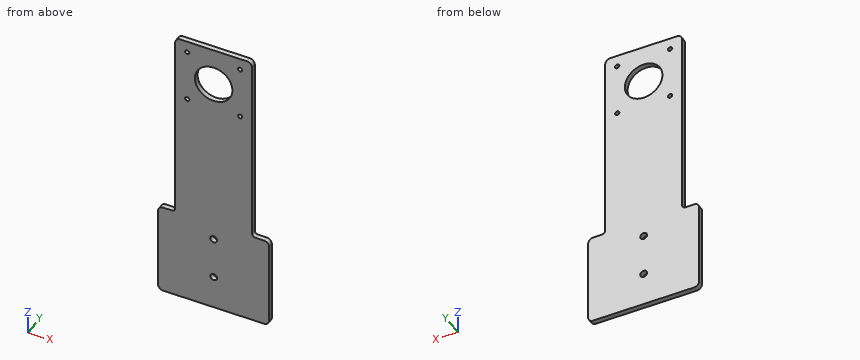
```python
from build123d import *

# Parameters (mm, degrees)
SKETCH1_R           = 2
SKETCH1_R_2         = 1.25
SKETCH1_R_3         = 11
BOSS_EXTRUDE1_DEPTH = 3
FILLET1_R           = 3
FILLET2_R           = 3
FILLET3_R           = 3
FILLET4_R           = 3
FILLET5_R           = 3
FILLET7_R           = 3
FILLET8_R           = 2
FILLET9_R           = 2


with BuildPart() as part:
    # Sketch1 → Boss-Extrude1 (new body)
    with BuildSketch(Plane(origin=(0, 0, 0), x_dir=(1, 0, 0), z_dir=(0, 1, 0))):
        Polygon((0, 111.61362417), (-32.5, 111.61362417), (-32.5, 56.61362417), (-22.5, 56.61362417), (-22.5, -58.38637583), (0, -58.38637583), (22.5, -58.38637583), (22.5, 56.61362417), (32.5, 56.61362417), (32.5, 111.61362417), align=None)
        with Locations(Location((0, 91.61362417, 0), (0, 0, 270))):
            Circle(SKETCH1_R, mode=Mode.SUBTRACT)
        with Locations(Location((0, 66.61362417, 0), (0, 0, 270))):
            Circle(SKETCH1_R, mode=Mode.SUBTRACT)
        with Locations(Location((-15.5, -20.454039675, 0), (0, 0, 270))):
            Circle(SKETCH1_R_2, mode=Mode.SUBTRACT)
        with Locations(Location((-15.5, -51.454039675, 0), (0, 0, 270))):
            Circle(SKETCH1_R_2, mode=Mode.SUBTRACT)
        with Locations(Location((15.5, -51.454039675, 0), (0, 0, 270))):
            Circle(SKETCH1_R_2, mode=Mode.SUBTRACT)
        with Locations(Location((15.5, -20.454039675, 0), (0, 0, 270))):
            Circle(SKETCH1_R_2, mode=Mode.SUBTRACT)
        with Locations(Location((0, -35.954039675, 0), (0, 0, 270))):
            Circle(SKETCH1_R_3, mode=Mode.SUBTRACT)
    extrude(amount=BOSS_EXTRUDE1_DEPTH)

    # Fillet1
    fillet1_edges = [part.edges().sort_by_distance(p)[0] for p in [
        (32.5, 1.5, -111.61362417),
    ]]
    fillet(fillet1_edges, radius=FILLET1_R)

    # Fillet2
    fillet2_edges = [part.edges().sort_by_distance(p)[0] for p in [
        (-32.5, 1.5, -111.61362417),
    ]]
    fillet(fillet2_edges, radius=FILLET2_R)

    # Fillet3
    fillet3_edges = [part.edges().sort_by_distance(p)[0] for p in [
        (-32.5, 1.5, -56.61362417),
    ]]
    fillet(fillet3_edges, radius=FILLET3_R)

    # Fillet4
    fillet4_edges = [part.edges().sort_by_distance(p)[0] for p in [
        (32.5, 1.5, -56.61362417),
    ]]
    fillet(fillet4_edges, radius=FILLET4_R)

    # Fillet5
    fillet5_edges = [part.edges().sort_by_distance(p)[0] for p in [
        (22.5, 1.5, 58.38637583),
    ]]
    fillet(fillet5_edges, radius=FILLET5_R)

    # Fillet7
    fillet7_edges = [part.edges().sort_by_distance(p)[0] for p in [
        (-22.5, 1.5, 58.38637583),
    ]]
    fillet(fillet7_edges, radius=FILLET7_R)

    # Fillet8
    fillet8_edges = [part.edges().sort_by_distance(p)[0] for p in [
        (-22.5, 1.5, -56.61362417),
    ]]
    fillet(fillet8_edges, radius=FILLET8_R)

    # Fillet9
    fillet9_edges = [part.edges().sort_by_distance(p)[0] for p in [
        (22.5, 1.5, -56.61362417),
    ]]
    fillet(fillet9_edges, radius=FILLET9_R)


solid = part.part
```
Here's how the part is built. I have some questions about the finished solid (model axes, mm). Coordinates: 2 decimals unless noted, no trailing zeros. Order: outer loops, then holes, each group sorted by start corner. A loop starts at its lowest first (then second) coordinate and runs counter-clockwise, first axis right, second up. Notation, with made-up numbers: M 50.25,54 L 96.25,54 A28 cw 96.25,76 Z; hole C 11,40.5 d3. An arc over 180 degrees is marked long. Answer as a JSON object with one key per item and string values. Group by question number.
(1) Suppose I cut it at B-B, the plane y = 0.9. Please give me the cut outline in (x, z), then the cut area to 3 significant figures.
(2) Suppose I cut it at A-A, the plane x = 0. Please give me the cut outline in (y, z), then the cut area to 3 significant figures.
(3) Suppose I cut it at C-C, the plane z = -22.5. Please give me the cut outline in (x, y).
(4) Suppose I cut it at D-D, the plane x = -26.5. Please give me the cut outline in (y, z).
(5) For pin 1 (5 mm diameter, centred on x = 21, z = -89, fed in from -Y); pin 2 (1.5 mm diameter, centred on y = 1, z = -41, fed in from +X); pin 3 (0.9 mm diameter, centred on x = -26, y = 1.5, fed in from +Z), each with a flat end and sliding along its axis, tell me the tip position at first contact or that it passes through.
(6) I need wall thicknesses on probe 1 along X at (y, z) = (0.65, 20.5); probe 2 along Z at (x, y) = (14.5, 1.05); probe 3 along X at (y, z) = (2.8, 52). Which ranges of each line are inside material? Lowest first, please.
Values found:
{
 "1": {"outline": "M -32.5,-108.61 A3 ccw -29.5,-111.61 L 29.5,-111.61 A3 ccw 32.5,-108.61 L 32.5,-59.61 A3 ccw 29.5,-56.61 L 24.5,-56.61 A2 cw 22.5,-54.61 L 22.5,55.39 A3 ccw 19.5,58.39 L -19.5,58.39 A3 ccw -22.5,55.39 L -22.5,-54.61 A2 cw -24.5,-56.61 L -29.5,-56.61 A3 ccw -32.5,-59.61 Z; hole C -15.5,20.45 d2.5; hole C -15.5,51.45 d2.5; hole C 0,35.95 d22; hole C 0,-91.61 d4; hole C 0,-66.61 d4; hole C 15.5,20.45 d2.5; hole C 15.5,51.45 d2.5", "area": "8,320 mm^2"},
 "2": {"outline": "M 0,-111.61 L 3,-111.61 L 3,-93.61 L 0,-93.61 Z; M 0,-89.61 L 3,-89.61 L 3,-68.61 L 0,-68.61 Z; M 0,-64.61 L 3,-64.61 L 3,24.95 L 0,24.95 Z; M 0,46.95 L 3,46.95 L 3,58.39 L 0,58.39 Z", "area": "420 mm^2"},
 "3": {"outline": "M -22.5,0 L 22.5,0 L 22.5,3 L -22.5,3 Z"},
 "4": {"outline": "M 0,-111.61 L 3,-111.61 L 3,-56.61 L 0,-56.61 Z"},
 "5": {"pin 1": "stops at y = 0", "pin 2": "stops at x = 22.5", "pin 3": "stops at z = -56.61"},
 "6": {"probe 1": "x = -22.5 to -16.75, -14.25 to 14.25, 16.75 to 22.5", "probe 2": "z = -111.61 to 19.7, 21.2 to 50.7, 52.2 to 58.39", "probe 3": "x = -22.5 to -16.62, -14.38 to 14.38, 16.62 to 22.5"}
}
